Geometry check sheet. Reference: the model listing, model coordinates, mm. Face numbers are marked on the shaded views. A direction names the side the tool comes from. Round coordinates to 2 decimals unless told otherwise and drop trailing zeros. Write each loop counter-clockwise with the first axis right and the second up, starting at its lowest first coordinate (ties: lowest second). Pieces come first, ordered by that corner, then holes. Notation, with made-up numbers: M 47,86.25 L 59,86.25 A23 ccw 59,120.25 Z; hole C 23,17.25 d8. An arc over 180 degrees is marked long. Answer as CSV lines item,"result". Start each with the question number.
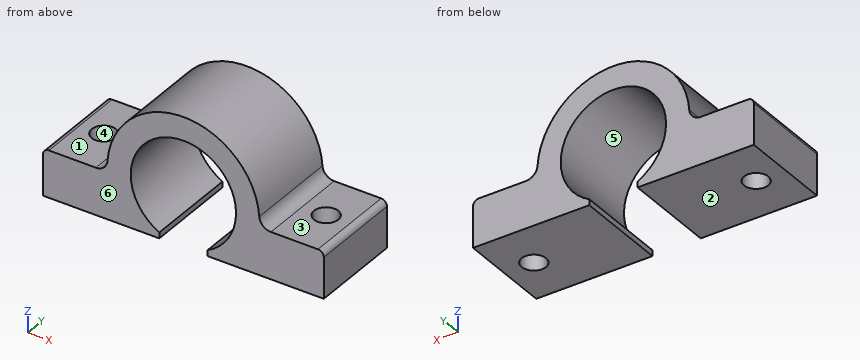
Autodesk Inventor part; units mm, degrees
ref_plane "YZ Plane" through (0, 0, 0) normal (1, 0, 0) x (0, 1, 0)
ref_plane "XZ Plane" through (0, 0, 0) normal (0, 1, 0) x (-1, 0, 0)
ref_plane "XY Plane" through (0, 0, 0) normal (0, 0, 1) x (1, 0, 0)
sketch "Sketch1" plane through (0, 0, 0) normal (0, 1, 0) x (-1, 0, 0)
  line L0 (0, 0) -> (38.1, 0)
  line L1 (38.1, 0) -> (38.1, 34.925)
  line L2 (38.1, 34.925) -> (0, 34.925)
  line L3 (0, 34.925) -> (0, 0)
  line L4 (19.05, 34.925) -> (19.05, 0) construction
  line L5 (-19.05, 12.7) -> (-19.05, 0)
  line L6 (-19.05, 0) -> (0, 0)
  line L7 (57.15, 12.7) -> (57.15, 0)
  line L8 (57.15, 0) -> (38.1, 0)
  line L9 (-19.05, 12.7) -> (0, 12.7)
  line L10 (38.1, 12.7) -> (57.15, 12.7)
  line L11 (0, 14.2875) -> (38.1, 14.2875) construction
  circle A0 centre (19.05, 14.2875) radius 14.2875
  line L12 (12.5046, 1.5875) -> (12.5046, 0)
  line L13 (25.5954, 1.5875) -> (25.5954, 0)
  arc A1 (39.6264, 12.7) -> (-1.5264, 12.7) centre (19.05, 14.2875) ccw
  point P0 (0, 22.225)
  point P1 (38.1, 22.225)
  dimension "d0" = 38.1
  dimension "d1" = 34.925
  dimension "d9" = 12.7
  dimension "d10" = 19.05
  dimension "d11" = 19.05
  dimension "d12" = 12.7
  dimension "d21" = 28.575
  dimension "d22" = 14.2875
  dimension "d34" = 1.5875
extrude "Extrusion1" add sketch "Sketch1" along normal blind 25.4 contours L3 A1 L1 L0 L13 A0 L12 | L6 L5 L9 L3 | L9 A1 L3 | L1 L10 L7 L8 | A1 L10 L1
fillet "Fillet1" radius 3.175 2 edges at (-39.6264, 12.7, 12.7) (1.5264, 12.7, 12.7)
fillet "Fillet1" radius 1.5875 2 edges at (19.05, 12.7, 12.7) (-57.15, 12.7, 12.7)
sketch "Sketch2" plane through (19.05, 25.4, 0) normal (0, 0, -1) x (-1, 0, 0)
  line L0 (14.3405, 0) -> (1.5875, 0) construction
  line L1 (74.6125, 0) -> (61.8595, 0) construction
  circle A0 centre (7.9375, -12.7) radius 3.302
  circle A1 centre (68.2625, -12.7) radius 3.302
  line L2 (74.6125, -25.4) -> (61.8595, -25.4)
  line L3 (14.3405, -25.4) -> (1.5875, -25.4)
  line L4 (74.6125, -25.4) -> (74.6125, 0) construction
  line L5 (1.5875, 0) -> (1.5875, -25.4) construction
  line L6 (0, -12.7) -> (76.2, -12.7) construction
  line L7 (38.1, 0) -> (38.1, -25.4) construction
  line L8 (23.8125, 0) -> (52.3875, 0)
  line L9 (23.8125, -25.4) -> (52.3875, -25.4)
  line L10 (0, -25.4) -> (0, 0)
  line L11 (76.2, -25.4) -> (76.2, 0)
  line L12 (61.8595, 0) -> (61.8595, -25.4)
  line L13 (14.3405, -25.4) -> (14.3405, 0)
  point P0 (31.5546, 0)
  point P1 (31.5546, -25.4)
  point P2 (38.1, 0)
  dimension "d15" = 6.604
  dimension "d16" = 6.604
  dimension "d24" = 30.1625
  dimension "d25" = 30.1625
  dimension "d26" = 60.325
extrude "Extrusion3" cut sketch "Sketch2" against normal through all
sketch "Sketch5" plane through (-25.5954, 0, 0) normal (0, 0, -1) x (-1, 0, 0)
  line L0 (-44.6454, 0) -> (-44.6454, 25.4)
  line L1 (31.5546, 0) -> (31.5546, 25.4)
  circle A0 centre (23.6171, 12.7) radius 3.302
  circle A1 centre (-36.7079, 12.7) radius 3.302
  line L2 (-44.6454, 25.4) -> (31.5546, 25.4)
  line L3 (-44.6454, 0) -> (31.5546, 0)
equation "\"d9\" = d12"
equation "\"d11\" = d10"
equation "\"d15\" = d16"
equation "\"d25\" = d24"
properties part number "Bearing Block V1.500 Drivetrain" material "Aluminum 6061"
1) Go/stop test with flat-tipped pins: pin 1 (4 mm diameter, centred on x = 13.5, y = 9.5, fed in from +Z); pin 2 (4 mm diameter, centred on y = 12.5, z = 25, fed in from -X); pin 3 (1.5 mm diameter, centred on y = 14, z = 19, fed in from +X); pin 4 (4 mm diameter, centred on x = -49.21, y = 12.7, fed in from +Z). Record where each tip stops, or that it passes through.
2) Section check A-A, the plane y = 12.7. Give the number of separate pieces and of enclosed holes in the cut face, plus the area to 3 significant figures.
3) Section check C-C, the plane x = -50. Record the cut outline in (y, z).
4) Scan lines: line 1 (X direction, y = 13.5, z = 8); line 2 (X direction, y = 13, z = 7); line 3 (Z direction, x = -27.5, y = 18.5). Record each from-to range of solid material in increasing order. Write a range as from..to.
5) Access from +Z, -Z, +X, -X, +Y, -Y to the whole of each face (thin tool, end or side, straight path). Record for the marked faces 1, 2 and 3.
6) Section check D-D, the plane z = 8.5. Record the cut outline in (x, y).
7) Section check B-B, the plane z = 26. Record the cut outline in (x, y).
8) Mould release check, pull along Y, two halves, no side actions. Record for the marked faces 4, 5 and 6: released by +Y, released by -Y, zero draft, split by the parting line, or undercut.
Results:
1,pin 1,"stops at z = 12.7"
1,pin 2,"stops at x = -37.76"
1,pin 3,"stops at x = 1.2"
1,pin 4,"passes through"
2,separate pieces,"3"
2,enclosed holes,"0"
2,area,"889 mm^2"
3,outline,"M 0,0 L 9.49,0 L 9.49,12.7 L 0,12.7 Z; M 15.91,0 L 25.4,0 L 25.4,12.7 L 15.91,12.7 Z"
4,line 1,"x = -57.15..-52.42, -46.01..-31.88, -6.22..7.91, 14.32..19.05"
4,line 2,"x = -57.15..-52.5, -45.92..-31.34, -6.76..7.82, 14.4..19.05"
4,line 3,"z = 0..2.77, 25.81..33.12"
5,face 1,"+Z, -X, +Y, -Y"
5,face 2,"-Z, +X, -X, +Y, -Y"
5,face 3,"+Z, +X, +Y, -Y"
6,outline,"M -57.15,0 L -32.11,0 L -32.11,25.4 L -57.15,25.4 Z; M -5.99,0 L 19.05,0 L 19.05,25.4 L -5.99,25.4 Z; hole C -49.21,12.7 d6.6; hole C 11.11,12.7 d6.6"
7,outline,"M -36.04,0 L -27.23,0 L -27.23,25.4 L -36.04,25.4 Z; M -10.87,0 L -2.06,0 L -2.06,25.4 L -10.87,25.4 Z"
8,face 4,"undercut"
8,face 5,"zero draft"
8,face 6,"released by -Y"
